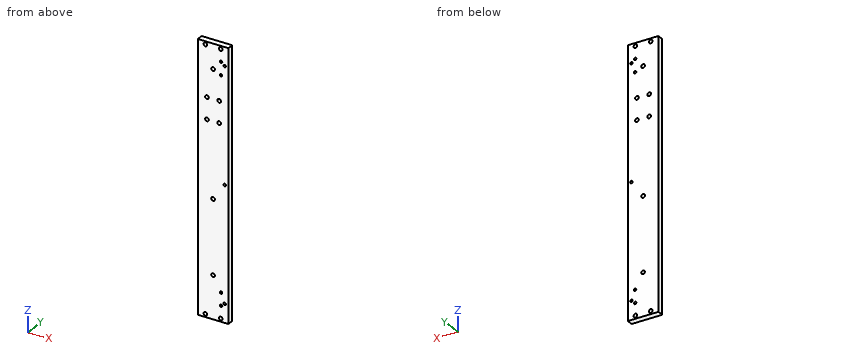
Autodesk Inventor part; units mm, degrees
ref_plane "YZ Plane" through (0, 0, 0) normal (1, 0, 0) x (0, 1, 0)
ref_plane "XZ Plane" through (0, 0, 0) normal (0, 1, 0) x (-1, 0, 0)
ref_plane "XY Plane" through (0, 0, 0) normal (0, 0, 1) x (1, 0, 0)
sketch "Boceto1" plane through (0, 0, 0) normal (0, 1, 0) x (-1, 0, 0)
  line L0 (22.6121, 129.278) -> (-27.3879, 129.278)
  line L1 (-27.3879, 129.278) -> (-27.3879, -304.722)
  line L2 (-27.3879, -304.722) -> (22.6121, -304.722)
  line L3 (22.6121, -304.722) -> (22.6121, 129.278)
  circle A0 centre (-15.3879, 104.278) radius 2
  circle A1 centre (-15.3879, 83.278) radius 2
  line L4 (-27.3879, -87.722) -> (-4.9043, -87.722)
  circle A2 centre (-15.3879, -279.722) radius 2
  circle A3 centre (-15.3879, -258.722) radius 2
  line L5 (-27.3879, -304.722) -> (-21.3879, -304.722)
  line L6 (-21.3879, -304.722) -> (-21.3879, -274.722)
  circle A4 centre (-21.3879, -274.722) radius 2
  circle A5 centre (-21.3879, -87.722) radius 2
  circle A6 centre (-21.3879, 99.278) radius 2
  circle A7 centre (-2.3879, -235.222) radius 3
  circle A8 centre (-2.3879, -115.222) radius 3
  circle A9 centre (-2.3879, 89.278) radius 3
  dimension "d4" = 434
  dimension "d5" = 50
  dimension "d16" = 4
  dimension "d17" = 4
  dimension "d18" = 25
  dimension "d19" = 21
  dimension "d20" = 12
  dimension "d21" = 12
  dimension "d85" = 12
  dimension "d86" = 12
  dimension "d87" = 21
  dimension "d89" = 30
  dimension "d90" = 4
  dimension "d91" = 4
  dimension "d92" = 44
  dimension "d93" = 44
  dimension "d94" = 217
  dimension "d95" = 6
  dimension "d96" = 25
  dimension "d97" = 69.5
  dimension "d98" = 6
  dimension "d99" = 120
  dimension "d100" = 25
  dimension "d101" = 6
  dimension "d102" = 25
  dimension "d103" = 40
extrude "Extrusión1" add sketch "Boceto1" along normal blind 10
sketch "Boceto2" plane through (0, 10, 0) normal (0, 1, 0) x (1, 0, 0)
  line L0 (-22.6121, -129.278) -> (27.3879, -129.278)
  line L1 (-22.6121, -129.278) -> (-22.6121, -124.278)
  line L2 (-22.6121, 304.722) -> (-22.6121, -129.278)
  line L3 (-22.6121, -124.278) -> (27.3879, -124.278)
  line L4 (27.3879, -129.278) -> (27.3879, 304.722)
  line L5 (27.3879, 304.722) -> (-22.6121, 304.722)
  line L6 (-22.6121, 304.722) -> (-22.6121, 299.722)
  line L7 (-22.6121, 299.722) -> (27.3879, 299.722)
  line L8 (-22.6121, -124.278) -> (-10.1121, -124.278)
  line L9 (27.3879, 299.722) -> (14.8879, 299.722)
  circle A0 centre (-10.1121, -124.278) radius 3
  circle A1 centre (14.8879, -124.278) radius 3
  circle A2 centre (-10.1121, 299.722) radius 3
  circle A3 centre (14.8879, 299.722) radius 3
  dimension "d6" = 5
  dimension "d7" = 5
  dimension "d8" = 12.5
  dimension "d9" = 12.5
  dimension "d10" = 6
  dimension "d11" = 6
  dimension "d12" = 6
  dimension "d13" = 6
  dimension "d30" = 5
  dimension "d74" = 5
extrude "Extrusión2" cut sketch "Boceto2" against normal blind 20 contours A0 L3 | L3 A0 | A1 L3 | L3 A1 | A2 L7 | L7 A2 | A3 L7 | L7 A3
thread "Thread1"
thread "Thread2"
sketch "Boceto3" plane through (0, 0, 0) normal (0, -1, 0) x (1, 0, 0)
  line L0 (27.3879, 129.278) -> (27.3879, -304.722)
  line L1 (12.3879, 42.078) -> (-7.6121, 42.078)
  line L2 (-7.6121, 42.078) -> (-7.6121, 7.078)
  line L3 (-7.6121, 7.078) -> (12.3879, 7.078)
  line L4 (12.3879, 7.078) -> (12.3879, 42.078)
  circle A0 centre (12.3879, 7.078) radius 3
  circle A1 centre (-7.6121, 7.078) radius 3
  circle A2 centre (12.3879, 42.078) radius 3
  circle A3 centre (-7.6121, 42.078) radius 3
  line L5 (-22.6121, 129.278) -> (27.3879, 129.278)
  line L6 (-22.6121, -304.722) -> (-22.6121, 129.278)
  point P0 (-14161.5164, 17179.1084)
  point P1 (-14161.5164, 17617.1084)
  point P2 (-14211.5164, 17617.1084)
  point P3 (-14211.5164, 17179.1084)
  dimension "d58" = 35
  dimension "d59" = 15
  dimension "d60" = 87.2
  dimension "d61" = 15
  dimension "d62" = 20
hole "Agujero1" at (12.3879, 0, 42.078) at (-7.6121, 0, 42.078) at (12.3879, 0, 7.078) at (-7.6121, 0, 7.078) direction (0, 1, 0) diameter 6 depth 12 tip angle 118
thread "Rosca5"
thread "Rosca6"
thread "Rosca7"
thread "Rosca8"
thread "Rosca9"
thread "Rosca10"
thread "Rosca11"
thread "Rosca12"
thread "Rosca13"
thread "Rosca14"
equation "\"d100\" = d96"
equation "\"d102\" = d96"
properties part number "Lateral" material "Aluminio 6061"
The listing builds one solid part. Answer for the finished solid, in the listing's coordinates (mm). Give positions to 0.01 mm unless a question says otherwise; leave off trailing zeros. One line per question, with ' | ' between items. Start each with the question number.
1. Section A-A, the plane y = 8 is taken. Count the separate pieces of the cut face and the enclosed holes in it, then the cut area to 3 significant figures.
2. Given P1, Ø9.5, axis at x = 14.89, z = -299.72, coming from the -Y side, flat-ended and moving along its own axis, determine where the tip first touches the part or whether it passes through.
3. Straight lines are drawn through the part: line 1 (Z direction, x = 21, y = 9.25); line 2 (Z direction, x = 20, y = 8); line 3 (Z direction, x = 11, y = 5.25). For each, find the intervals that lie inside material, in ascending order.
Result:
1) separate pieces: 1 | enclosed holes: 18 | area: 21,300 mm2
2) P1: stops at y = 0
3) line 1: z = -304.72 to -276.68, -272.76 to -89.68, -85.76 to 97.32, 101.24 to 129.28 | line 2: z = -304.72 to -276.16, -273.28 to -89.16, -86.28 to 97.84, 100.72 to 129.28 | line 3: z = -304.72 to 4.42, 9.74 to 39.42, 44.74 to 129.28
